Read the model definition and answer for the solid it produces. Units are mm, in the model's axes. Face numbers are marked on the shaded views. A direction names the side the tool comes from. Give positions to 0.01 mm unless a question says otherwise; leave off trailing zeros. Write each loop counter-clockwise with the first axis right and the second up, starting at its lowest first coordinate (ties: lowest second). Pieces come first, ordered by that corner, then holes. Notation, with made-up numbers: M -39.75,65.25 L -2.75,65.25 A23 cw -2.75,85.25 Z; hole C -19.75,88.25 d6. An arc over 180 degrees is marked long. Put each result on its own line as item: value.
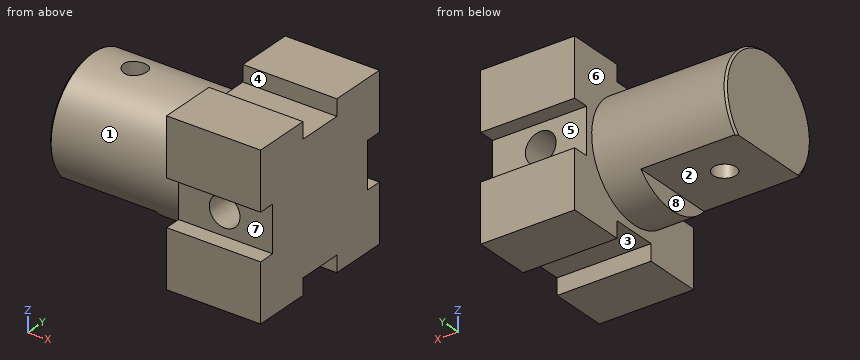
Autodesk Inventor part; units mm, degrees
ref_plane "YZ Plane" through (0, 0, 0) normal (1, 0, 0) x (0, 1, 0)
ref_plane "XZ Plane" through (0, 0, 0) normal (0, 1, 0) x (-1, 0, 0)
ref_plane "XY Plane" through (0, 0, 0) normal (0, 0, 1) x (1, 0, 0)
sketch "Эскиз1" plane through (0, 0, 0) normal (0, 0, 1) x (1, 0, 0)
  line L0 (-12.25, -21) -> (12.25, -21)
  line L1 (12.25, -21) -> (12.25, 21)
  line L2 (12.25, 21) -> (-12.25, 21)
  line L3 (-12.25, 21) -> (-12.25, -21)
  line L4 (-12.25, -21) -> (12.25, 21) construction
  line L5 (12.25, -21) -> (-12.25, 21) construction
  point P0 (0, 0)
  dimension "d0" = 24.5
  dimension "d1" = 42
extrude "Выдавливание1" add sketch "Эскиз1" along normal mid plane 42
sketch "Эскиз2" plane through (-12.25, -21, 21) normal (-1, 0, 0) x (0, 0, 1)
  circle A0 centre (-21, 21) radius 15
  dimension "d4" = 30
extrude "Выдавливание2" add sketch "Эскиз2" along normal blind 35
sketch "Эскиз3" plane through (-47.25, 0, 0) normal (-1, 0, 0) x (0, 0, 1)
  circle A0 centre (0, 0) radius 15
  line L0 (-10, -11.1803) -> (-10, 11.1803)
  dimension "d7" = 25
extrude "Выдавливание3" cut sketch "Эскиз3" against normal blind 25 contours L0 A0 picked at (-11.6306, -0.5993)
chamfer "Фаска1" distance 0.5 angle 45 2 edges at (-47.25, -13.6931, 6.1237) (-47.25, 13.6931, 6.1237)
sketch "Эскиз4" plane through (-12.25, 21, 21) normal (0, 1, 0) x (1, 0, 0)
  line L0 (24.5, 42) -> (24.5, 0)
  line L1 (0, 15) -> (24.5, 15)
  line L2 (24.5, 15) -> (24.5, 27)
  line L3 (24.5, 27) -> (0, 27)
  line L4 (0, 27) -> (0, 15)
  line L5 (0, 15) -> (24.5, 27) construction
  line L6 (24.5, 15) -> (0, 27) construction
  point P0 (12.25, 21)
  dimension "d13" = 12
extrude "Выдавливание4" cut sketch "Эскиз4" against normal blind 4.25
sketch "Эскиз5" plane through (-12.25, -21, 21) normal (0, -1, 0) x (1, 0, 0)
  line L0 (24.5, -42) -> (24.5, 0)
  line L1 (0, -15) -> (24.5, -15)
  line L2 (24.5, -15) -> (24.5, -27)
  line L3 (24.5, -27) -> (0, -27)
  line L4 (0, -27) -> (0, -15)
  line L5 (0, -15) -> (24.5, -27) construction
  line L6 (24.5, -15) -> (0, -27) construction
  point P0 (12.25, -21)
  dimension "d16" = 12
extrude "Выдавливание5" cut sketch "Эскиз5" against normal blind 4.25
sketch "Эскиз6" plane through (0, 0, -21) normal (0, 0, -1) x (-1, 0, 0)
  line L0 (-12.25, -21) -> (-12.25, 21)
  line L1 (12.25, 6) -> (-12.25, 6)
  line L2 (-12.25, 6) -> (-12.25, -6)
  line L3 (-12.25, -6) -> (12.25, -6)
  line L4 (12.25, -6) -> (12.25, 6)
  line L5 (12.25, 6) -> (-12.25, -6) construction
  line L6 (-12.25, 6) -> (12.25, -6) construction
  point P0 (0, 0)
  dimension "d19" = 12
extrude "Выдавливание6" cut sketch "Эскиз6" against normal blind 4.25
sketch "Эскиз7" plane through (0, 0, 21) normal (0, 0, 1) x (1, 0, 0)
  line L0 (-12.25, 6) -> (-12.25, -6)
  line L1 (12.25, 6) -> (-12.25, 6)
  line L2 (-12.25, 6) -> (-12.25, -6)
  line L3 (-12.25, -6) -> (12.25, -6)
  line L4 (12.25, -6) -> (12.25, 6)
  line L5 (12.25, 6) -> (-12.25, -6) construction
  line L6 (-12.25, 6) -> (12.25, -6) construction
  point P0 (0, 0)
  dimension "d22" = 12
extrude "Выдавливание7" cut sketch "Эскиз7" against normal blind 4.25
sketch "Эскиз8" plane through (-22.25, -11.1803, -10) normal (0, 0, -1) x (-1, 0, 0)
  line L0 (25, 21.6803) -> (25, 0.6803)
  point P0 (-22.25, 11.1803)
  point P1 (13.6, 11.1803)
  dimension "d25" = 11.4
hole "Отверстие1" at (-35.85, 0, -10) direction (0, 0, 1) diameter 6 end through all
sketch "Эскиз9" plane through (-12.25, 16.75, 21) normal (0, 1, 0) x (1, 0, 0)
  line L0 (24.5, 27) -> (24.5, 15)
  point P0 (12.25, 21)
  point P1 (12, 21)
  dimension "d33" = 12.5
hole "Отверстие2" at (-0.25, 16.75, 0) direction (0, -1, 0) diameter 8 end through all
(1) Section C-C on x = -0.25 is taken. Determine the outline of the cut face in (y, z), and give its area (3 significant figures).
Result:
outline: M -21,-21 L -6,-21 L -6,-16.75 L 6,-16.75 L 6,-21 L 21,-21 L 21,-6 L 16.75,-6 L 16.75,-4 L -16.75,-4 L -16.75,-6 L -21,-6 Z; M -21,6 L -16.75,6 L -16.75,4 L 16.75,4 L 16.75,6 L 21,6 L 21,21 L 6,21 L 6,16.75 L -6,16.75 L -6,21 L -21,21 Z
area: 1,290 mm²
(2) Section D-D on y = 17.5 is taken. Determine the outline of the cut face in (x, z), and give its area (3 significant figures).
Result:
outline: M -12.25,-21 L 12.25,-21 L 12.25,-6 L -12.25,-6 Z; M -12.25,6 L 12.25,6 L 12.25,21 L -12.25,21 Z
area: 735 mm²
(3) Section A-A on z = 0 is taken. Determine the outline of the cut face in (x, y).
Result:
outline: M -47.25,-14.5 L -46.75,-15 L -12.25,-15 L -12.25,-16.75 L -4.25,-16.75 L -4.25,16.75 L -12.25,16.75 L -12.25,15 L -46.75,15 L -47.25,14.5 Z; M 3.75,-16.75 L 12.25,-16.75 L 12.25,16.75 L 3.75,16.75 Z; hole C -35.85,0 d6
(4) Section B-B on y = 0 is taken. Determine the outline of the cut face in (x, z).
Result:
outline: M -47.25,-10 L -38.85,-10 L -38.85,15 L -46.75,15 L -47.25,14.5 Z; M -32.85,-10 L -22.25,-10 L -22.25,-15 L -12.25,-15 L -12.25,-16.75 L 12.25,-16.75 L 12.25,16.75 L -12.25,16.75 L -12.25,15 L -32.85,15 Z; hole C -0.25,0 d8
(5) For a pull along Y with two mould halves and no side action, classify the marked faces 1, 2 and 3 as +Y half, -Y half, draft (parallel to the pull), parting line (faces both ways), or undercut.
Result:
face 1: parting line
face 2: draft
face 3: undercut
(6) Given pin 1 Ø4 at (x, z) = (-37.5, -4.5) entering from +Y; pin 2 Ø10 at (x, z) = (3.5, -3) entering from +Y; pin 3 Ø3 at (x, y) = (-20.5, 1.5) entering from -Z; pin 4 Ø8 at (x, y) = (-35.85, 0) entering from +Z, each flat-ended and moving along its own axis, determine where each tip first touches the part or whether it passes through.
Result:
pin 1: stops at y = 14.79
pin 2: stops at y = 21
pin 3: stops at z = -15
pin 4: stops at z = 15
(7) Which of the six approach directions +Z, -Z, +X, -X, +Y, -Y give full straight-line access (tool end or side, diameter ignored) to the marked faces 4, 5, 6, 7 and 8?
Result:
face 4: +Z, +X, -X
face 5: +X, -X, +Y
face 6: -X
face 7: +X, -X, -Y
face 8: -Z, -X, +Y, -Y
(8) Straight lines are drawn through the part: line 1 along X through (y, z) = (-8.5, 0); line 2 along X through (y, z) = (-2, 2.5); line 3 along Y through (x, z) = (1, -19). For each, find the intervals that lie inside material, in ascending order. Write a range as from..to.
Result:
line 1: x = -47.25..-4.25, 3.75..12.25
line 2: x = -47.25..-38.09, -33.61..-3.37, 2.87..12.25
line 3: y = -21..-6, 6..21
